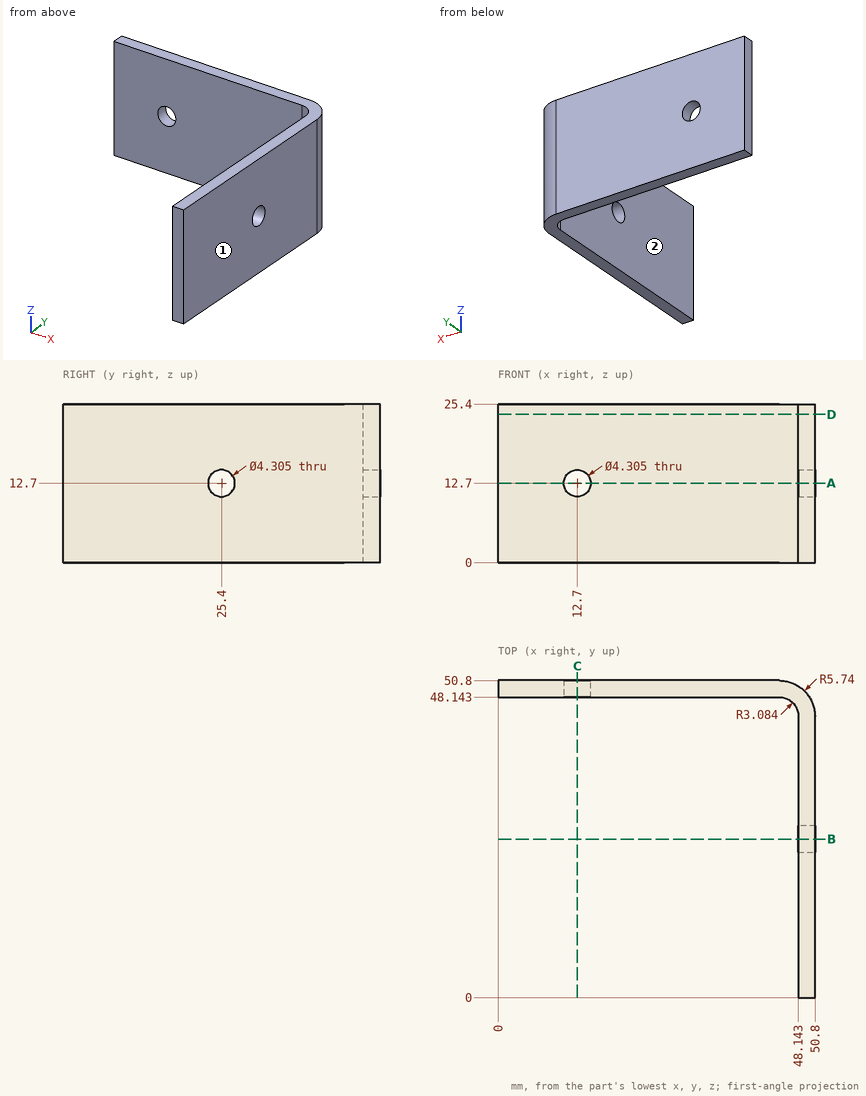
Check sheet for the drawn part. Datum: minimum x, y, z corner. Units: mm. A direction names the side the tool comes from. Round coordinates to 2 decimals unless told otherwise and drop trailing zeros. Order: outer loops, then holes, each group sorted by start corner. A loop starts at its lowest first (then second) coordinate and runs counter-clockwise, first axis right, second up.
1) Tool access check on the marked faces 1 and 2. Record the directions out of +Z, -Z, +X, -X, +Y, -Y that give a thin tool (end or side, any length) a straight path to the whole face; none if there is none.
2) Section check A-A (z = 12.7). Record the boundary of the cut face in (x, y), and give its area (3 significant figures).
3) Section check D-D (z = 23.75). Record the boundary of the cut face in (x, y), and give its area (3 significant figures).
4) Go/stop test with flat-tipped pins: pin 1 Ø6 at (y, z) = (15, 17) entering from -X; pin 2 Ø4 at (x, z) = (12.7, 12.7) entering from -Y; pin 3 Ø4 at (x, z) = (34.5, 19.5) entering from -Y. Record where each tip stops, or that it passes through.
5) Section check B-B (y = 25.4). Record the boundary of the cut face in (x, z).
6) Scan lines: line 1 (Z direction, x = 49.4, y = 25.4); line 2 (X direction, y = 37, z = 6.5). Record each from-to range of solid material in increasing order.
Result:
1. face 1: +Z, -Z, +X, +Y, -Y
1. face 2: +Z, -Z, -X, -Y
2. outline: (0, 48.14) - (10.55, 48.14) - (10.55, 50.8) - (0, 50.8) - close; (14.85, 48.14) - (45.06, 48.14) arc R3.08 cw to (48.14, 45.06) - (48.14, 27.55) - (50.8, 27.55) - (50.8, 45.06) arc R5.74 ccw to (45.06, 50.8) - (14.85, 50.8) - close; (48.14, 0) - (50.8, 0) - (50.8, 23.25) - (48.14, 23.25) - close
2. area: 235 mm2
3. outline: (0, 48.14) - (45.06, 48.14) arc R3.08 cw to (48.14, 45.06) - (48.14, 0) - (50.8, 0) - (50.8, 45.06) arc R5.74 ccw to (45.06, 50.8) - (0, 50.8) - close
3. area: 258 mm2
4. pin 1: stops at x = 48.14
4. pin 2: passes through
4. pin 3: stops at y = 48.14
5. outline: (48.14, 0) - (50.8, 0) - (50.8, 10.55) - (48.14, 10.55) - close; (48.14, 14.85) - (50.8, 14.85) - (50.8, 25.4) - (48.14, 25.4) - close
6. line 1: z = 0 to 10.55, 14.85 to 25.4
6. line 2: x = 48.14 to 50.8
